Could you check a few things on this drawing? It's one solid part, dimensions in mm from its lowest x, y, z. A direction names the side the tool comes from. Coordinates: 2 decimals unless noted, no trailing zeros. Loops run counter-clockwise (first coordinate to the right, second up) from the corner with the lowest first, then second, coordinate; pieces in that order, holes last. Notation, with made-up numbers: (-33, 5.5) -> (25, 5.5) arc R25 ccw to (25, 42.5) -> close; hole circle Ø8 at (54.5, -7.75). An arc over 180 degrees is marked (long way). One line per question, with ' | ' between items.
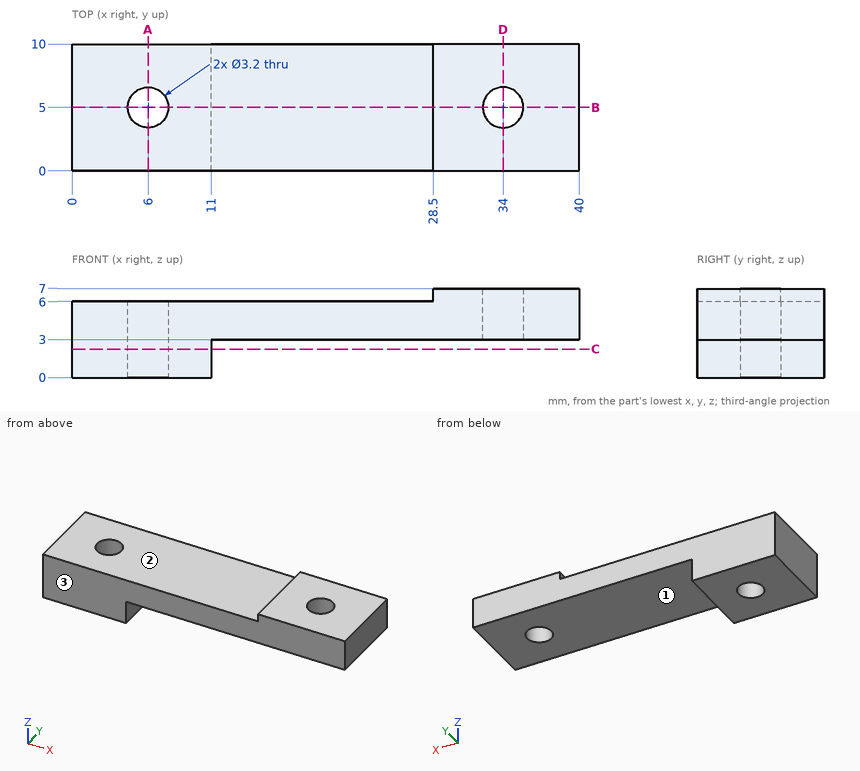
1) I need wall thicknesses on line 1 along Y through (x, z) = (34, 5.3); line 2 along Z through (x, y) = (16.5, 5); line 3 along X through (y, z) = (4.5, 4.75). Which ranges of each line are inside material? Lowest first, please. Write a range as from..to.
Data:
line 1: 0..3.4, 6.6..10 | line 2: 3..6 | line 3: 0..4.48, 7.52..32.48, 35.52..40
2) If we section it at A-A on x = 6: Please give me the cut outline in (y, z), and give its area (3 significant figures).
Data:
outline: (0, 0) -> (3.4, 0) -> (3.4, 6) -> (0, 6) -> close; (6.6, 0) -> (10, 0) -> (10, 6) -> (6.6, 6) -> close | area: 40.8 mm²
3) If we section it at C-C on z = 2.25: Please give me the cut outline in (x, y), and give its area (3 significant figures).
Data:
outline: (0, 0) -> (11, 0) -> (11, 10) -> (0, 10) -> close; hole circle Ø3.2 at (6, 5) | area: 102 mm²
4) I'm going to push flat-ended pins straight in: pin 1 Ø1 at (x, y) = (23.5, 8.5) entering from -Z; pin 2 Ø1.5 at (x, y) = (20.5, 9) entering from +Z. Where does each tip first touch, or does it pass through?
Data:
pin 1: z = 3 | pin 2: z = 6
5) On a 3-axis mill with a long thin cutter (end or side, diameter ignored), from which of +Z, -Z, +X, -X, +Y, -Y can I reach the whole of each face in a straight line? I mean the marked faces 1, 2 and 3. Say none if no direction works.
Data:
face 1: -Z, +X, +Y, -Y | face 2: +Z, -X, +Y, -Y | face 3: +Z, -Z, +X, -X, -Y
6) If we section it at B-B on y = 5: Please give me the cut outline in (x, z), and give its area (4 significant figures).
Data:
outline: (0, 0) -> (4.4, 0) -> (4.4, 6) -> (0, 6) -> close; (7.6, 0) -> (11, 0) -> (11, 3) -> (32.4, 3) -> (32.4, 7) -> (28.5, 7) -> (28.5, 6) -> (7.6, 6) -> close; (35.6, 3) -> (40, 3) -> (40, 7) -> (35.6, 7) -> close | area: 132.5 mm²
7) If we section it at D-D on x = 34: Please give me the cut outline in (y, z).
Data:
outline: (0, 3) -> (3.4, 3) -> (3.4, 7) -> (0, 7) -> close; (6.6, 3) -> (10, 3) -> (10, 7) -> (6.6, 7) -> close
